Can you work these out from the drawing? Everything is in mm from the part's minimum corner. A direction names the side the tool comes from. Give positions to 0.01 mm unless a question says otherwise; leave off trailing zeros. Loops run counter-clockwise (first coordinate to the right, second up) from the corner with the lowest first, then second, coordinate; pieces in that order, holes last. Notation, with made-up numbers: M 73,23.5 L 117,23.5 A36 cw 117,57.5 Z; hole C 18,86.25 d2. An arc over 180 degrees is marked long. Use CSV: the item, a comma, the result in double quotes.
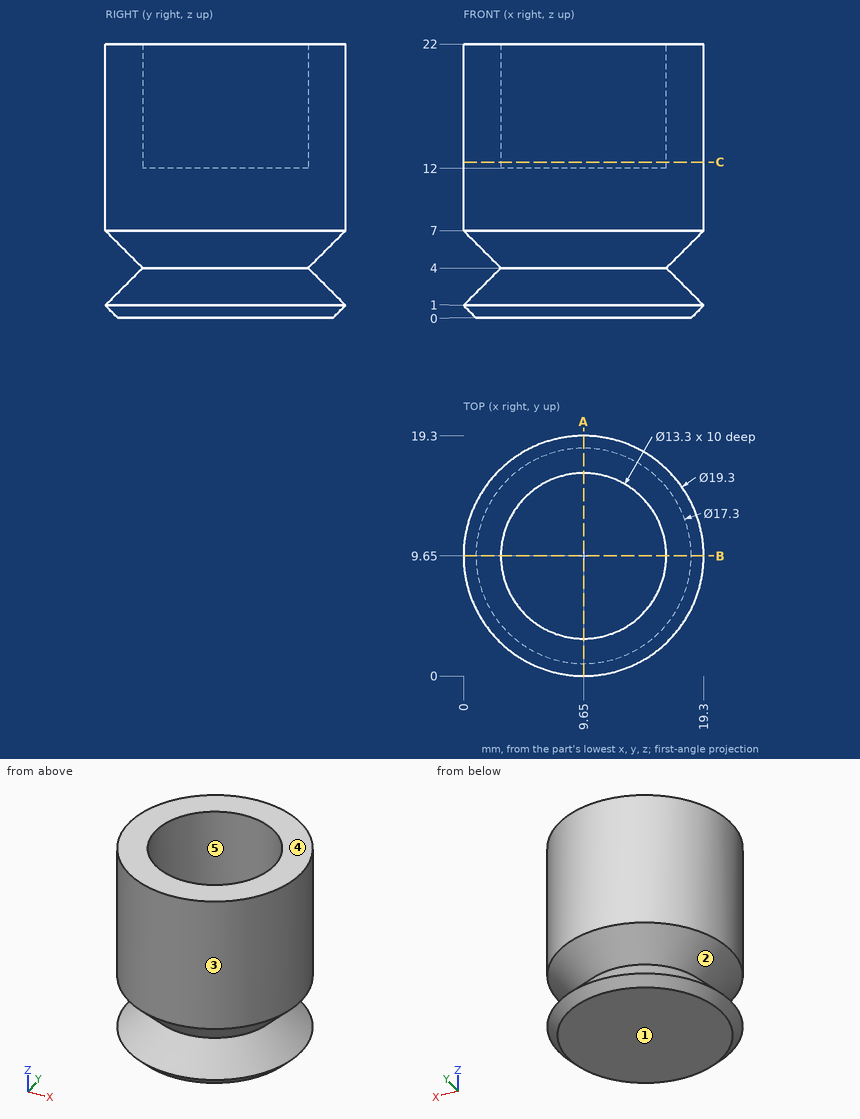
Q1. If we mould it in two halves opening along Y, with no side actions, what happens to the marked faces 3, 4 and 5? For each: released by +Y, released by -Y, zero draft, split by the parting line, or undercut.
Model answer:
face 3,"split by the parting line"
face 4,"zero draft"
face 5,"undercut"
Q2. For the marked faces 1 and 2, which set-ups out of +Z, -Z, +X, -X, +Y, -Y let a thin tool reach every point of the face, with its end or its side?
Model answer:
face 1,"-Z, +X, -X, +Y, -Y"
face 2,"none"
Q3. I want a section at A-A, the plane x = 9.65. Please give me the cut outline in (y, z), then the cut area to 3 significant figures.
Model answer:
outline,"M 0,1 L 1,0 L 18.3,0 L 19.3,1 L 16.3,4 L 19.3,7 L 19.3,22 L 16.3,22 L 16.3,12 L 3,12 L 3,22 L 0,22 L 0,7 L 3,4 Z"
area,"273 mm2"
Q4. Please list where these lines run through material, in increasing order: L1, parallel to Y at x = 9.65, z = 17.25; L2, parallel to Z at x = 1.5, y = 6.5; L3, parallel to Z at x = 12.25, y = 17.25. Write a range as from..to.
Model answer:
L1,"0..3, 16.3..19.3"
L2,"0.09..1.91, 6.09..22"
L3,"0..2.62, 5.38..22"
Q5. I'm going to push flat-ended pins straight in: P1, Ø1.5, axis at x = 14, z = 18, coming from the +Y side; P2, Ø1.5, axis at x = 13.5, z = 5, coming from the +Y side; P3, Ø8, axis at y = 14.5, z = 19, coming from the -X side. Where does each tip first touch, or does it pass through?
Model answer:
P1,"y = 18.6"
P2,"y = 17.19"
P3,"x = 0.04"
Q6. I want a section at C-C, the plane z = 12.5. Please give me the cut outline in (x, y).
Model answer:
outline,"C 9.65,9.65 d19.3; hole C 9.65,9.65 d13.3"
